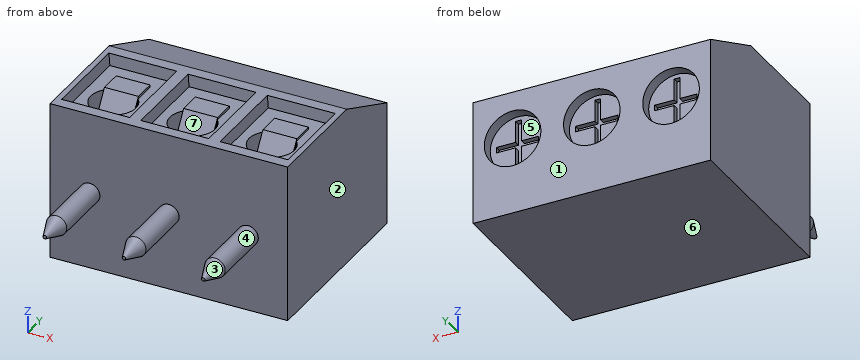
```python
from build123d import *

# Parameters (mm, degrees)
BOSS_EXTRUDE1_DEPTH         = 10.5
SKETCH2_R                   = 1.25
CUT_EXTRUDE1_DEPTH          = 0.5
SKETCH3_W                   = 3
SKETCH3_H                   = 4
CUT_EXTRUDE2_DEPTH          = 0.5
CUT_EXTRUDE2_TAPER          = 10
SKETCH4_R                   = 1
CUT_EXTRUDE3_DEPTH          = 6
SKETCH6_R                   = 0.45
BOSS_EXTRUDE3_DEPTH         = 3.8
CHAMFER1_SIZE               = 1
CHAMFER1_SIZE2              = 0.371896666
EXTRUDE_THIN1_DEPTH         = 0.75
SKETCH8_W                   = 0.25
SKETCH8_H                   = 2.158330758
SKETCH8_W_2                 = 1.874325027
SKETCH8_H_2                 = 0.25
CUT_EXTRUDE_THIN1_DEPTH     = 0.25
LPATTERN1_COUNT             = 3
LPATTERN1_PITCH             = 3.5
CHAMFER1_OF_LPATTERN1_SIZE2 = 0.371896666
CHAMFER1_OF_LPATTERN1_SIZE  = 1


with BuildPart() as part:
    # Sketch1 → Boss-Extrude1 (new body)
    with BuildSketch(Plane(origin=(0, 0, 0), x_dir=(0, 0, -1), z_dir=(1, 0, 0))):
        Polygon((0, 5), (1.5, 8.4), (7, 8.4), (7, 0), (0, 0), align=None)
    extrude(amount=BOSS_EXTRUDE1_DEPTH)

    # Sketch2 → Cut-Extrude1 (cut)
    with BuildSketch(Plane(origin=(0, 8.4, 0), x_dir=(1, 0, 0), z_dir=(0, 1, 0))):
        with Locations((1.75, 3.6)):
            Circle(SKETCH2_R)
    cut_extrude1 = extrude(amount=-CUT_EXTRUDE1_DEPTH, mode=Mode.SUBTRACT)

    # Sketch3 → Cut-Extrude2 (cut)
    with BuildSketch(Plane.XY):
        with Locations((1.75, 2.5)):
            Rectangle(SKETCH3_W, SKETCH3_H)
    cut_extrude2 = extrude(amount=-CUT_EXTRUDE2_DEPTH, taper=CUT_EXTRUDE2_TAPER, mode=Mode.SUBTRACT)

    # Sketch4 → Cut-Extrude3 (cut)
    with BuildSketch(Plane.XY.offset(-0.5)):
        with Locations((1.75, 2)):
            Circle(SKETCH4_R)
    cut_extrude3 = extrude(amount=-CUT_EXTRUDE3_DEPTH, mode=Mode.SUBTRACT)

    # Sketch6 → Boss-Extrude3 (add)
    with BuildSketch(Plane.XZ):
        with Locations((1.75, -3.6)):
            Circle(SKETCH6_R)
    boss_extrude3 = extrude(amount=BOSS_EXTRUDE3_DEPTH)

    # Chamfer1
    chamfer1_edges = [part.edges().sort_by_distance(p)[0] for p in [
        (1.3, -3.8, -3.6),
    ]]
    chamfer1_side = [part.faces().sort_by_distance(p)[0] for p in [
        (1.3, -1.9, -3.6),
    ]]
    chamfer(chamfer1_edges, length=CHAMFER1_SIZE, length2=CHAMFER1_SIZE2, reference=chamfer1_side[0])

    # Sketch7 → Extrude-Thin1 (add, symmetric)
    with BuildSketch(Plane(origin=(1.75, 0, 0), x_dir=(0, 0, -1), z_dir=(1, 0, 0))):
        Polygon((0.5, 3.678716588), (0.5, 2.743158903), (1.89970396, 1.832221158), (5.88813409, 1.438302133), (5.878305368, 1.338786324), (1.865601336, 1.735102771), (0.4, 2.688927019), (0.4, 3.678716588), align=None)
    extrude_thin1 = extrude(amount=EXTRUDE_THIN1_DEPTH, both=True)

    # Sketch8 → Cut-Extrude-Thin1 (cut, symmetric)
    with BuildSketch(Plane(origin=(0, 7.9, 0), x_dir=(1, 0, 0), z_dir=(0, 1, 0))):
        with Locations((1.75, 3.611637798)):
            Rectangle(SKETCH8_W, SKETCH8_H)
        with Locations((1.795143175, 3.611637798)):
            Rectangle(SKETCH8_W_2, SKETCH8_H_2)
    cut_extrude_thin1 = extrude(amount=CUT_EXTRUDE_THIN1_DEPTH, both=True, mode=Mode.SUBTRACT)

    # LPattern1: Cut-Extrude1, Cut-Extrude2, Cut-Extrude3, Boss-Extrude3, Extrude-Thin1, Cut-Extrude-Thin1 ×3
    with Locations(*[(i * LPATTERN1_PITCH, 0, 0) for i in range(1, LPATTERN1_COUNT)]):
        add(cut_extrude1, mode=Mode.SUBTRACT)
        add(cut_extrude2, mode=Mode.SUBTRACT)
        add(cut_extrude3, mode=Mode.SUBTRACT)
        add(boss_extrude3)
        add(extrude_thin1)
        add(cut_extrude_thin1, mode=Mode.SUBTRACT)

    # Chamfer1 of LPattern1
    chamfer1_of_lpattern1_edges = [part.edges().sort_by_distance(p)[0] for p in [
        (4.8, -3.8, -3.6),
        (8.3, -3.8, -3.6),
    ]]
    chamfer(chamfer1_of_lpattern1_edges, length=CHAMFER1_OF_LPATTERN1_SIZE, length2=CHAMFER1_OF_LPATTERN1_SIZE2)


solid = part.part
```
CAD build for the part. Positions are in the model's coordinates, mm. Face numbers are marked on the shaded views. A direction names the side the tool comes from. Coordinates: 2 decimals unless noted, no trailing zeros. Write each loop counter-clockwise with the first axis right and the second up, starting at its lowest first coordinate (ties: lowest second). Pieces come first, ordered by that corner, then holes. Notation, with made-up numbers: (-15.5, 11) -> (-2.5, 11) arc R25 ccw to (-2.5, 50) -> close; hole circle Ø5 at (67.25, 25). An arc over 180 degrees is marked (long way). Return JSON: item names as keys, results as strings. Group by question number.
Q1. Cut at C-C, the plane z = -4.5. State how many separate pieces and enclosed holes the cut face has, then the cut area to 3 significant figures.
Q2. Which spindle directions (+Z, -Z, +X, -X, +Y, -Y) get a long thin tool onto all of the face, cutting with end or side? Do the marked faces 4, 5, 6 and 7. Say none if no direction does.
Q3. Cut at B-B, the plane y = -1.75. Give the cut face in (x, z), then the cut area to 3 significant figures.
Q4. Cut at A-A, the plane z = -5.5. Give the cut face in (x, y).
Q5. Drill centre lines: line 1 (X direction, y = 2, z = -5); line 2 (X direction, y = 8.1, z = -3.6); line 3 (Y direction, x = 4, z = -5.5). Where is each one in solid material? Low to high.
Q6. Pull direction X, two halves, no side cores. Call the marked faces 1, 2 and 3: released by +X, released by -X, zero draft, split by the parting line, or undercut.
Q7. Flat gauge pins, fed straight in: pin 1 (3 mm diameter, centred on x = 1.5, y = 5, fed in from +Z); pin 2 (4 mm diameter, centred on x = 5, z = -1, fed in from -Y). Where does each tip first touch, or does it go through?
Returned:
{
 "1": {"separate pieces": "4", "enclosed holes": "3", "area": "76.4 mm2"},
 "2": {"face 4": "-Y", "face 5": "+Y", "face 6": "-Z, +X, -X, +Y, -Y", "face 7": "+Z"},
 "3": {"outline": "circle Ø0.9 at (1.75, -3.6); circle Ø0.9 at (5.25, -3.6); circle Ø0.9 at (8.75, -3.6)", "area": "1.91 mm2"},
 "4": {"outline": "(0, 0) -> (10.5, 0) -> (10.5, 8.4) -> (0, 8.4) -> close; (1, 1.38) -> (2.5, 1.38) -> (2.5, 1.48) -> (1, 1.48) -> close; (4.5, 1.38) -> (6, 1.38) -> (6, 1.48) -> (4.5, 1.48) -> close; (8, 1.38) -> (9.5, 1.38) -> (9.5, 1.48) -> (8, 1.48) -> close; hole circle Ø2 at (1.75, 2); hole circle Ø2 at (5.25, 2); hole circle Ø2 at (8.75, 2)"},
 "5": {"line 1": "x = 0 to 0.75, 2.75 to 4.25, 6.25 to 7.75, 9.75 to 10.5", "line 2": "x = 0 to 0.5, 3 to 4, 6.5 to 7.5, 10 to 10.5", "line 3": "y = 0 to 8.4"},
 "6": {"face 1": "zero draft", "face 2": "released by +X", "face 3": "undercut"},
 "7": {"pin 1": "stops at z = 0", "pin 2": "stops at y = 0"}
}
